For this review, use the dimensioned drawing (mm, ordinates from the lowest corner) and the shaded views. A direction names the side the tool comes from. Round coordinates to 2 decimals unless told otherwise and drop trailing zeros. Write each loop counter-clockwise with the first axis right and the second up, starting at its lowest first coordinate (ties: lowest second). Pieces come first, ordered by that corner, then holes.
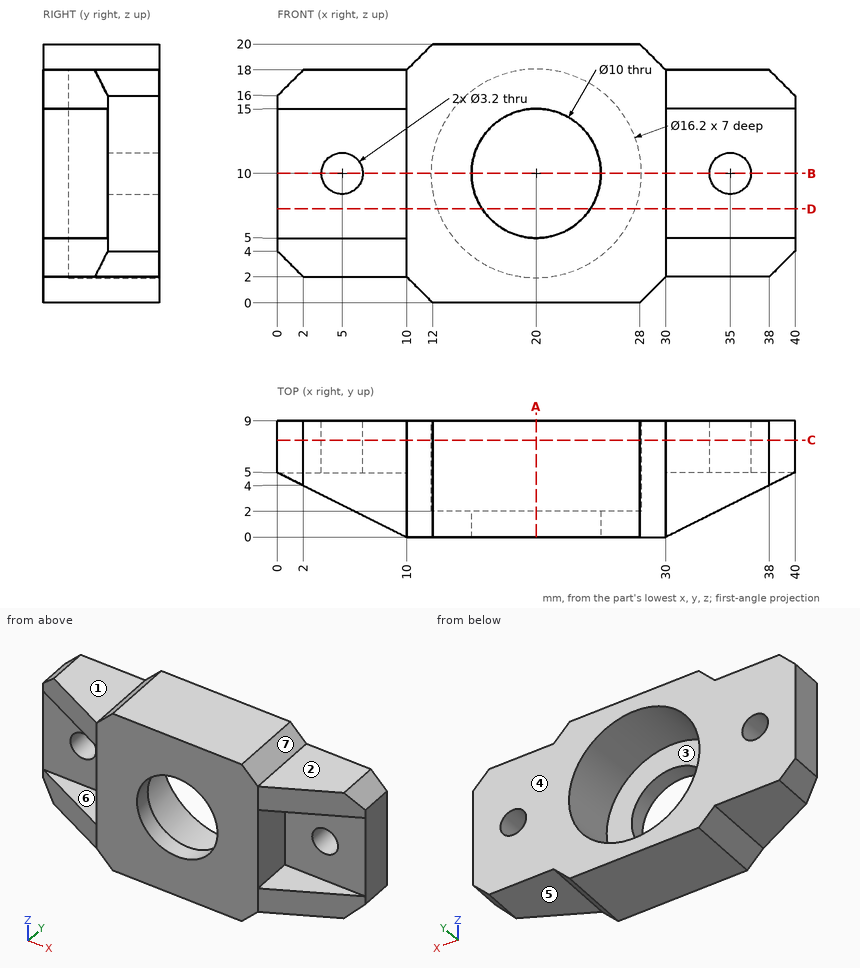
(1) For pin 1 Ø4 at (x, y) = (7, 2.5) entering from +Z; pin 2 Ø1.5 at (y, z) = (1.5, 11.5) entering from -X; pin 3 Ø2 at (x, z) = (5, 7) entering from -Y, all flat-tipped, find the tip position at first contact; note any pin that passes through.
Geometry check:
pin 1: stops at z = 18
pin 2: stops at x = 10
pin 3: stops at y = 5
(2) For line 1 along X through (y, z) = (8.2, 10); line 2 along X through (y, z) = (3.5, 10); line 3 along Z through (x, y) = (5, 6.35), list the stretches that pass through material, from the lowest coordinate up.
Geometry check:
line 1: x = 0 to 3.4, 6.6 to 11.9, 28.1 to 33.4, 36.6 to 40
line 2: x = 10 to 11.9, 28.1 to 30
line 3: z = 2 to 8.4, 11.6 to 18
(3) We need section C-C, the plane y = 7.5. Give the boundary of the cut face in (x, z).
Geometry check:
outline: (0, 4) - (2, 2) - (10, 2) - (12, 0) - (28, 0) - (30, 2) - (38, 2) - (40, 4) - (40, 16) - (38, 18) - (30, 18) - (28, 20) - (12, 20) - (10, 18) - (2, 18) - (0, 16) - close; hole circle Ø3.2 at (5, 10); hole circle Ø16.2 at (20, 10); hole circle Ø3.2 at (35, 10)
(4) We need section A-A, the plane x = 20. Give the boundary of the cut face in (y, z), and give its area (3 significant figures).
Geometry check:
outline: (0, 0) - (9, 0) - (9, 1.9) - (2, 1.9) - (2, 5) - (0, 5) - close; (0, 15) - (2, 15) - (2, 18.1) - (9, 18.1) - (9, 20) - (0, 20) - close
area: 46.6 mm2
(5) Mouldability with a two-part tool opening along Z and no side actions: class the marked faces 4, 5, 6 and 7 as pulls with the +Z half, pulls with the -Z half, needs draft (parallel to the pull), parting line crosses it, or undercut.
Geometry check:
face 4: needs draft
face 5: pulls with the -Z half
face 6: undercut
face 7: pulls with the +Z half
(6) We need section D-D, the plane z = 7.25. Give the boundary of the cut face in (x, y), and give its area (3 significant figures).
Geometry check:
outline: (0, 5) - (10, 5) - (10, 0) - (15.82, 0) - (15.82, 2) - (12.38, 2) - (12.38, 9) - (0, 9) - close; (24.18, 0) - (30, 0) - (30, 5) - (40, 5) - (40, 9) - (27.62, 9) - (27.62, 2) - (24.18, 2) - close
area: 137 mm2
(7) For the marked faces 1, 2 and 3, list the 3-axis set-ups (+Z, -Z, +X, -X, +Y, -Y) from which the entire face can be reached by the end or side of a thin tool; tool diameter is ignored.
Geometry check:
face 1: +Z, -X, +Y, -Y
face 2: +Z, +X, +Y, -Y
face 3: +Y
(8) We need section B-B, the plane z = 10. Give the boundary of the cut face in (x, y), and give its area (3 significant figures).
Geometry check:
outline: (0, 5) - (3.4, 5) - (3.4, 9) - (0, 9) - close; (6.6, 5) - (10, 5) - (10, 0) - (15, 0) - (15, 2) - (11.9, 2) - (11.9, 9) - (6.6, 9) - close; (25, 0) - (30, 0) - (30, 5) - (33.4, 5) - (33.4, 9) - (28.1, 9) - (28.1, 2) - (25, 2) - close; (36.6, 5) - (40, 5) - (40, 9) - (36.6, 9) - close
area: 101 mm2
